Here's how the part is built. I have some questions about the finished solid (model axes, mm). Face numbers are marked on the shaded views. A direction names the side the tool comes from. Coordinates: 2 decimals unless noted, no trailing zeros. Order: outer loops, then holes, each group sorted by start corner. A loop starts at its lowest first (then second) coordinate and runs counter-clockwise, first axis right, second up. Notation, with made-up numbers: (14, 39.5) - (54, 39.5) arc R22 ccw to (54, 72.5) - close; hole circle Ø2 at (-34, 75.5). An arc over 180 degrees is marked (long way). Answer in a Markdown table with one row per item. Add a question column.
Item 1: Thinking about a two-plate mould opening in Y: for the marked faces 1, 2 and 3, which applies, +Y half, -Y half, draft (parallel to the pull), parting line (faces both ways), or undercut?
Item 2: On a 3-axis mill with a long thin cutter (end or side, diameter ignored), from which of +Z, -Z, +X, -X, +Y, -Y can I reach the whole of each face in a straight line? I mean the marked faces 4, 5 and 6. Say none if no direction works.
Item 3: I want a section at C-C (y = 49.5). Please give me the cut outline in (x, z), plus the area to 3 significant figures.
Item 4: I want a section at D-D (y = 18). Please give me the cut outline in (x, z).
Item 5: I want a section at B-B (z = 5). Please give me the cut outline in (x, y), plus the area to 3 significant figures.
Item 6: If I drill on line 1 along Z through (x, y) = (23, 101); line 2 along Y through (x, z) = (-3, 10); line 3 along X through (y, z) = (7.75, 32.5), over which ranges is the centre line in solid material (lowest first)? Write a range as from..to.
Item 7: Will these pins go through, and if not, where does the flat tip stop? pin 1 Ø2 at (y, z) = (29.5, 16.5) entering from -X; pin 2 Ø1.5 at (x, z) = (7.5, 32) entering from -Y; pin 3 Ø8.5 at (x, z) = (2.5, 32) entering from -Y.
Item 8: I want a section at A-A (z = 13.5). Please give me the cut outline in (x, y).
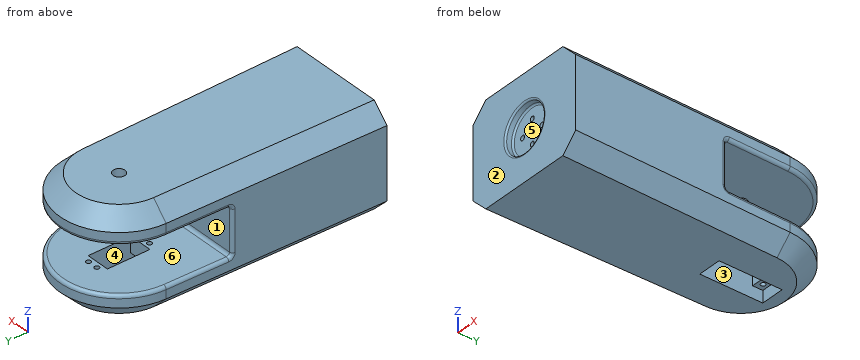
```python
from build123d import *

# Parameters (mm, degrees)
BOSS_EXTRUDE1_DEPTH = 65
CHAMFER1_SIZE       = 10
SKETCH2_R           = 15
CUT_EXTRUDE1_DEPTH  = 5
SKETCH4_R           = 1.5
CUT_EXTRUDE2_DEPTH  = 7.5
FILLET1_R           = 1
SKETCH5_W           = 30
SKETCH5_H           = 78
CUT_EXTRUDE3_DEPTH  = 44.75
FILLET2_R           = 2
SKETCH6_W           = 15
SKETCH6_H           = 40
CUT_EXTRUDE4_DEPTH  = 7.5
SKETCH7_W           = 15
SKETCH7_H           = 27
SKETCH7_R           = 1.5
CUT_EXTRUDE5_DEPTH  = 10
SKETCH8_R           = 3.75
CUT_EXTRUDE6_DEPTH  = 191.918831033


with BuildPart() as part:
    # Sketch1 → Boss-Extrude1 (new body)
    with BuildSketch(Plane.XY):
        with BuildLine():
            Line((-40, 0), (40, 0))
            Line((40, 0), (37.493833718, 138.180024354))
            ThreePointArc((37.493833718, 138.180024354), (0, 175), (-37.493833718, 138.180024354))
            Line((-37.493833718, 138.180024354), (-40, 0))
        make_face()
    extrude(amount=BOSS_EXTRUDE1_DEPTH)

    # Chamfer1
    chamfer1_edges = [part.edges().sort_by_distance(p)[0] for p in [
        (-38.746916859, 69.090012177, 65),
        (38.746916859, 69.090012177, 65),
        (-38.746916859, 69.090012177, 0),
        (0, 175, 0),
        (38.746916859, 69.090012177, 0),
        (0, 175, 65),
    ]]
    chamfer(chamfer1_edges, length=CHAMFER1_SIZE)

    # Sketch2 → Cut-Extrude1 (cut)
    with BuildSketch(Plane(origin=(0, 0, 0), x_dir=(-1, 0, 0), z_dir=(0, -1, 0))):
        with Locations(Location((0, -32.5, 0), (0, 0, 90))):
            Circle(SKETCH2_R)
    extrude(amount=-CUT_EXTRUDE1_DEPTH, mode=Mode.SUBTRACT)

    # Sketch4 → Cut-Extrude2 (cut)
    with BuildSketch(Plane.XZ.offset(-5)):
        with Locations(Location((0, 40, 0), (0, 0, 270))):
            Circle(SKETCH4_R)
        with Locations(Location((7.5, 32.5, 0), (0, 0, 270))):
            Circle(SKETCH4_R)
        with Locations(Location((0, 25, 0), (0, 0, 270))):
            Circle(SKETCH4_R)
        with Locations(Location((-7.5, 32.5, 0), (0, 0, 270))):
            Circle(SKETCH4_R)
    extrude(amount=-CUT_EXTRUDE2_DEPTH, mode=Mode.SUBTRACT)

    # Fillet1
    fillet1_edges = [part.edges().sort_by_distance(p)[0] for p in [
        (0, 5, 47.5),
        (0, 0, 47.5),
    ]]
    fillet(fillet1_edges, radius=FILLET1_R)

    # Sketch5 → Cut-Extrude3 (cut, symmetric)
    with BuildSketch(Plane(origin=(0, 0, 0), x_dir=(0, 0, -1), z_dir=(1, 0, 0))):
        with Locations((-32.5, 136)):
            Rectangle(SKETCH5_W, SKETCH5_H)
    extrude(amount=CUT_EXTRUDE3_DEPTH, both=True, mode=Mode.SUBTRACT)

    # Fillet2
    fillet2_edges = [part.edges().sort_by_distance(p)[0] for p in [
        (-38.240714383, 97, 32.5),
        (-37.867274051, 117.590012177, 47.5),
        (-37.867274051, 117.590012177, 17.5),
        (0, 97, 17.5),
        (37.867274051, 117.590012177, 17.5),
        (0, 175, 17.5),
        (0, 175, 47.5),
        (37.867274051, 117.590012177, 47.5),
        (0, 97, 47.5),
        (38.240714383, 97, 32.5),
    ]]
    fillet(fillet2_edges, radius=FILLET2_R)

    # Sketch6 → Cut-Extrude4 (cut)
    with BuildSketch(Plane(origin=(0, 0, 0), x_dir=(-1, 0, 0), z_dir=(0, 0, -1))):
        with Locations((0, 137.5)):
            Rectangle(SKETCH6_W, SKETCH6_H)
    extrude(amount=-CUT_EXTRUDE4_DEPTH, mode=Mode.SUBTRACT)

    # Sketch7 → Cut-Extrude5 (cut)
    with BuildSketch(Plane(origin=(0, 0, 7.5), x_dir=(-1, 0, 0), z_dir=(0, 0, -1))):
        with Locations((0, 137.5)):
            Rectangle(SKETCH7_W, SKETCH7_H)
        with Locations(Location((-3.25, 154.25, 0), (0, 0, 90))):
            Circle(SKETCH7_R)
        with Locations(Location((3.25, 154.25, 0), (0, 0, 90))):
            Circle(SKETCH7_R)
        with Locations(Location((-3.25, 120.75, 0), (0, 0, 90))):
            Circle(SKETCH7_R)
        with Locations(Location((3.25, 120.75, 0), (0, 0, 90))):
            Circle(SKETCH7_R)
    extrude(amount=-CUT_EXTRUDE5_DEPTH, mode=Mode.SUBTRACT)

    # Sketch8 → Cut-Extrude6 (cut, through all)
    with BuildSketch(Plane(origin=(0, 0, 0), x_dir=(-1, 0, 0), z_dir=(0, 0, -1))):
        with Locations((0, 137.5)):
            Circle(SKETCH8_R)
    extrude(amount=-CUT_EXTRUDE6_DEPTH, mode=Mode.SUBTRACT)


solid = part.part
```
Values follow:
| question | item | result |
|---|---|---|
| 1 | face 1 | +Y half |
| 1 | face 2 | -Y half |
| 1 | face 3 | undercut |
| 2 | face 4 | -Z |
| 2 | face 5 | -Y |
| 2 | face 6 | +X, -X, +Y |
| 3 | outline | (-39.1, 10) - (-29.1, 0) - (29.1, 0) - (39.1, 10) - (39.1, 55) - (29.1, 65) - (-29.1, 65) - (-39.1, 55) - close |
| 3 | area | 4,880 mm^2 |
| 4 | outline | (-39.67, 10) - (-29.67, 0) - (29.67, 0) - (39.67, 10) - (39.67, 55) - (29.67, 65) - (-29.67, 65) - (-39.67, 55) - close |
| 5 | outline | (-35, 0) - (35, 0) - (32.49, 138.09) arc R32.5 ccw to (-32.49, 138.09) - close; hole (-7.5, 117.5) - (7.5, 117.5) - (7.5, 157.5) - (-7.5, 157.5) - close |
| 5 | area | 10,300 mm^2 |
| 6 | line 1 | z = 0..17.5, 47.5..65 |
| 6 | line 2 | y = 0..119.27, 122.23..124, 151..152.77, 155.73..174.88 |
| 6 | line 3 | x = -39.86..-9, -6..6, 9..39.86 |
| 7 | pin 1 | stops at x = -39.48 |
| 7 | pin 2 | stops at y = 12.5 |
| 7 | pin 3 | stops at y = 5 |
| 8 | outline | (-40, 0) - (40, 0) - (37.49, 138.18) arc R37.5 ccw to (-37.49, 138.18) - close; hole (-7.5, 124) - (7.5, 124) - (7.5, 151) - (-7.5, 151) - close; hole circle Ø3 at (-3.25, 120.75); hole circle Ø3 at (-3.25, 154.25); hole circle Ø3 at (3.25, 120.75); hole circle Ø3 at (3.25, 154.25) |
